The listing builds one solid part. Answer for the finished solid, in the listing's coordinates (mm). Face numbers are marked on the shaded views. A direction names the side the tool comes from. Round coordinates to 2 decimals unless told otherwise and drop trailing zeros. Order: outer loops, then holes, each group sorted by start corner. A loop starts at its lowest first (then second) coordinate and runs counter-clockwise, first axis right, second up. Notation, with made-up numbers: (40.5, 2) -> (99.5, 2) arc R28 cw to (99.5, 33) -> close; hole circle Ø9 at (10.5, 31). An arc over 180 degrees is marked (long way). Return JSON: item names as keys, results as strings. Group by question number.
(1) Which of the six approach directions +Z, -Z, +X, -X, +Y, -Y give full straight-line access (tool end or side, diameter ignored) to the marked faces 1 and 2?
(2) The part is cut by section A-A (y = 8). Determine the outline of the cut face in (x, z), plus the area to 3 significant figures.
(3) Consider line 1 (X direction, y = 8.5, z = 0.75); line 2 (Z direction, x = -3.25, y = 6); line 3 (Y direction, x = 5.75, z = -19.25). Determine where each line is inside the solid, lowest interval first. Write a range as [from, to].
(4) The part is cut by section C-C (x = -3.75). Determine the outline of the cut face in (y, z).
(5) Each of these flat-tipped pins is pushed along its axis until it touches: pin 1 (1.1 mm diameter, centred on x = -5.5, z = -14.5, fed in from +Y); pin 2 (2 mm diameter, centred on x = 0, y = -9.5, fed in from +Z); pin 3 (1.5 mm diameter, centred on x = -2.5, z = -16, fed in from +Y). Where does it stop, or does it pass through?
(6) Determine the mould class of the marked faces 3, 4, 5 and 6 for opening direction Y: +Y half, -Y half, draft (parallel to the pull), parting line (faces both ways), or undercut.
(7) The part is cut by section D-D (y = 4.5). Determine the outline of the cut face in (x, z), plus the area to 3 significant figures.
(8) The part is cut by section B-B (z = -19.5). Determine the outline of the cut face in (x, y).
Autodesk Inventor part; units mm, degrees
ref_plane "YZ Plane" through (0, 0, 0) normal (1, 0, 0) x (0, 1, 0)
ref_plane "XZ Plane" through (0, 0, 0) normal (0, 1, 0) x (-1, 0, 0)
ref_plane "XY Plane" through (0, 0, 0) normal (0, 0, 1) x (1, 0, 0)
sketch "Sketch1" plane through (0, 0, 0) normal (1, 0, 0) x (0, 1, 0)
  line L0 (0, 8) -> (0, 0)
  line L1 (0, 8) -> (15, 8)
  line L2 (15, 8) -> (15, 0)
  line L3 (6, 0) -> (6, 8) construction
  line L4 (0, 0) -> (15, 0)
  dimension "d38" = 6
  dimension "d40" = 8
  dimension "d59" = 15
extrude "Extrusion1" add sketch "Sketch1" along normal mid plane 12
sketch "Sketch3" plane through (6, 0, 8) normal (0, 0, 1) x (1, 0, 0)
  circle A0 centre (-6, 6) radius 3.05
  line L0 (-12, 0) -> (0, 0)
  line L1 (0, 15) -> (0, 0)
  circle A1 centre (-6, 9) radius 3.05
  line L2 (-2.95, 9) -> (-2.95, 6)
  line L3 (-9.05, 9) -> (-9.05, 6)
  point P0 (0, -6)
  dimension "d9" = 6.1
  dimension "d23" = 6
  dimension "d41" = 6
  dimension "d60" = 6.1
  dimension "d61" = 3
extrude "Extrusion3" cut sketch "Sketch3" against normal through all
sketch "Sketch8" plane through (-6, 0, 8) normal (0, 0, 1) x (1, 0, 0)
  arc A0 (2.95, 6) -> (9.05, 6) centre (6, 6) ccw construction
  circle A1 centre (6, 6) radius 5.5
  line L0 (0, 15) -> (0, 0)
  line L1 (0, 3) -> (1.3902, 3)
  line L2 (10.6098, 3) -> (12, 3)
  line L3 (12, 15) -> (12, 0)
  line L4 (12, 0) -> (12, -3)
  line L5 (12, -3) -> (0, -3)
  line L6 (0, -3) -> (0, 0)
  line L7 (0, 0) -> (12, 0) construction
  point P0 (6, 0)
  point P1 (12, 12.26)
  dimension "d47" = 11
  dimension "d48" = 6
  dimension "d49" = 3
extrude "Extrusion7" add sketch "Sketch8" against normal blind 30 contours A1 L2 L3 L4 L5 L6 L0 L1
sketch "Sketch9" plane through (-6, 0, -22) normal (0, 0, -1) x (-1, 0, 0)
  line L0 (-6.979, -3) -> (-6, -17)
  line L1 (-6, -17) -> (-5.021, -3)
  line L2 (-12, -3) -> (0, -3)
  line L3 (-6, -17) -> (-6, -3) construction
  point P0 (-6, 0)
  dimension "d54" = 14
  dimension "d55" = 4
  dimension "d56" = 4
extrude "Extrusion8" add sketch "Sketch9" against normal blind 8
equation "\"d56\" = d55"
properties part number "angle_pointer"
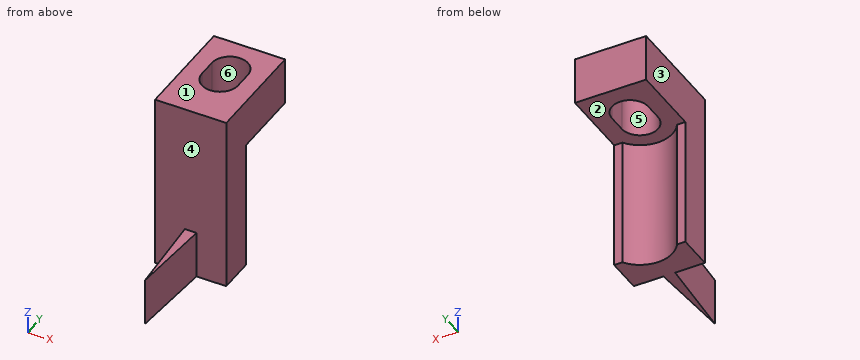
Answer below:
{
 "1": {"face 1": "+Z, +X, -X, +Y, -Y", "face 2": "-Z, +Y"},
 "2": {"outline": "(-6, 0) -> (-3.05, 0) -> (-3.05, 8) -> (-6, 8) -> close; (3.05, 0) -> (6, 0) -> (6, 8) -> (3.05, 8) -> close", "area": "47.2 mm²"},
 "3": {"line 1": "x = [-6, -3.05], [3.05, 6]", "line 2": "z = [0, 8]", "line 3": "y = [-3, 3]"},
 "4": {"outline": "(-3, -22) -> (1.98, -22) -> (1.98, 0) -> (15, 0) -> (15, 8) -> (-3, 8) -> close"},
 "5": {"pin 1": "stops at y = 3", "pin 2": "stops at z = -14", "pin 3": "stops at y = 1.56"},
 "6": {"face 3": "draft", "face 4": "-Y half", "face 5": "undercut", "face 6": "undercut"},
 "7": {"outline": "(-6, 0) -> (-2.66, 0) -> (-2.66, 8) -> (-6, 8) -> close; (2.66, 0) -> (6, 0) -> (6, 8) -> (2.66, 8) -> close", "area": "53.5 mm²"},
 "8": {"outline": "(-6, -3) -> (-0.98, -3) -> (0, -17) -> (0.98, -3) -> (6, -3) -> (6, 3) -> (4.61, 3) arc R5.5 cw to (-4.61, 3) -> (-6, 3) -> close"}
}
